Read the model definition and answer for the solid it produces. Units are mm, in the model's axes. A direction names the side the tool comes from. Give positions to 0.01 mm unless a question says otherwise; leave off trailing zeros. Return JSON: item names as keys, results as strings.
```python
from build123d import *
from OCP.BRepFilletAPI import BRepFilletAPI_MakeChamfer

# Parameters (mm, degrees)
BOSS_EXTRUDE1_DEPTH     = 27
SKETCH2_W               = 339
SKETCH2_H               = 271
CUT_EXTRUDE1_DEPTH      = 2.54
FILLET2_R               = 0.254
ESQUISSE1_W             = 314
ESQUISSE1_H             = 295.992698065
BOSS_EXTRU_1_DEPTH      = 25
CHANFREIN1_SIZE         = 25
CHANFREIN1_SIZE_2       = 35
ENL_V_MAT_EXTRU_1_DEPTH = 25
ESQUISSE3_R             = 2.5
ENL_V_MAT_EXTRU_2_DEPTH = 15


with BuildPart() as part:
    # Sketch1 → Boss-Extrude1 (new body)
    with BuildSketch(Plane.XY):
        with BuildLine():
            Line((9.729828387, -0.262968335), (184.729828387, -4.992698065))
            ThreePointArc((184.729828387, -4.992698065), (185, -4.996348366), (185.270171613, -4.992698065))
            Line((185.270171613, -4.992698065), (360.270171613, -0.262968335))
            ThreePointArc((360.270171613, -0.262968335), (367.165951302, 2.758487678), (370, 9.733381364))
            Line((370, 9.733381364), (370, 340))
            Line((370, 340), (0, 340))
            Line((0, 340), (0, 9.733381364))
            ThreePointArc((0, 9.733381364), (2.834048698, 2.758487678), (9.729828387, -0.262968335))
        make_face()
    extrude(amount=BOSS_EXTRUDE1_DEPTH)

    # Sketch2 → Cut-Extrude1 (cut)
    with BuildSketch(Plane.XY.offset(27)):
        with Locations((185, 184.5)):
            Rectangle(SKETCH2_W, SKETCH2_H)
    extrude(amount=-CUT_EXTRUDE1_DEPTH, mode=Mode.SUBTRACT)

    # Fillet2
    fillet2_edges = [part.edges().sort_by_distance(p)[0] for p in [
        (354.5, 184.5, 24.46),
        (15.5, 184.5, 27),
        (185, 49, 27),
        (185, 320, 27),
    ]]
    fillet(fillet2_edges, radius=FILLET2_R)

    # Esquisse1 → Boss.-Extru.1 (add)
    with BuildSketch(Plane(origin=(0, 0, 0), x_dir=(-1, 0, 0), z_dir=(0, 0, -1))):
        with Locations((-185, 155.003650967)):
            Rectangle(ESQUISSE1_W, ESQUISSE1_H)
    extrude(amount=BOSS_EXTRU_1_DEPTH)

    # Chanfrein1
    chanfrein1_edges_1 = [part.edges().sort_by_distance(p)[0] for p in [
        (28, 155.003650968, -25),
    ]]
    chanfrein1_side_1 = [part.faces().sort_by_distance(p)[0] for p in [
        (28, 155.003650968, -24.5),
    ]]
    chanfrein1_edges_2 = [part.edges().sort_by_distance(p)[0] for p in [
        (185, 303, -25),
    ]]
    chanfrein1_side_2 = [part.faces().sort_by_distance(p)[0] for p in [
        (185, 303, -24.5),
    ]]
    chanfrein1_edges_3 = [part.edges().sort_by_distance(p)[0] for p in [
        (342, 155.003650968, -25),
    ]]
    chanfrein1_side_3 = [part.faces().sort_by_distance(p)[0] for p in [
        (342, 155.003650968, -24.5),
    ]]
    chanfrein1 = BRepFilletAPI_MakeChamfer(part.part.solid().wrapped)
    for e in chanfrein1_edges_1:
        chanfrein1.Add(CHANFREIN1_SIZE - 0.0001, CHANFREIN1_SIZE_2 - 0.0001, e.wrapped, chanfrein1_side_1[0].wrapped)
    for e in chanfrein1_edges_2:
        chanfrein1.Add(CHANFREIN1_SIZE - 0.0001, CHANFREIN1_SIZE_2 - 0.0001, e.wrapped, chanfrein1_side_2[0].wrapped)
    for e in chanfrein1_edges_3:
        chanfrein1.Add(CHANFREIN1_SIZE - 0.0001, CHANFREIN1_SIZE_2 - 0.0001, e.wrapped, chanfrein1_side_3[0].wrapped)
    add(Compound.cast(chanfrein1.Shape()), mode=Mode.REPLACE)  # a hair under: the kernel refuses the full size

    # Esquisse2 → Enlèv. mat.-Extru.1 (cut)
    with BuildSketch(Plane(origin=(0, 0, -25), x_dir=(-1, 0, 0), z_dir=(0, 0, -1))):
        Polygon((-273.063305356, 7.007301935), (-89.826670404, 7.007301935), (-89.826670404, 60.007301935), (-66.826670404, 60.007301935), (-66.826670404, 108.007301935), (-296.063305356, 108.007301935), (-296.063305356, 60.007301935), (-273.063305356, 60.007301935), align=None)
    extrude(amount=-ENL_V_MAT_EXTRU_1_DEPTH, mode=Mode.SUBTRACT)

    # Esquisse3 → Enlèv. mat.-Extru.2 (cut)
    with BuildSketch(Plane(origin=(0, 0, -25), x_dir=(-1, 0, 0), z_dir=(0, 0, -1))):
        with Locations((-188, 255.8)):
            Circle(ESQUISSE3_R)
        with Locations((-238, 193)):
            Circle(ESQUISSE3_R)
        with Locations((-132, 193)):
            Circle(ESQUISSE3_R)
    extrude(amount=-ENL_V_MAT_EXTRU_2_DEPTH, mode=Mode.SUBTRACT)


solid = part.part
```
Q1. Consider L1, parallel to X at y = 193, z = -19.25; L2, parallel to X at y = 193, z = -19; L3, parallel to Y at x = 282, z = -19. Determine where each line is inside the solid, lowest interval first.
Values:
{"L1": "x = 54.95 to 129.5, 134.5 to 235.5, 240.5 to 315.05", "L2": "x = 54.6 to 129.5, 134.5 to 235.5, 240.5 to 315.4", "L3": "y = 7.01 to 60.01, 108.01 to 276.4"}
Q2. Determine the mould class of faces 5 (the flat face through (296.063, 84, -13)), 6 (the flat face through (300, 7.007, -12)), 7 (the flat face through (273.063, 34, -13)), 8 (the flat face through (183, 186, 24.46)) for opening direction Y: released by +Y, released by -Y, zero draft, split by the parting line, or undercut.
Values:
{"face 5": "undercut", "face 6": "released by -Y", "face 7": "zero draft", "face 8": "undercut"}
Q3. Given pin 1 (3 mm diameter, centred on x = 253, z = -18, fed in from +Y); pin 2 (3 mm diameter, centred on x = 187.5, z = -13, fed in from +Y); pin 3 (5 mm diameter, centred on x = 164.5, y = 305.5, fed in from +Z), each flat-ended and moving along its own axis, determine where each tip first touches the part or whether it passes through.
Values:
{"pin 1": "stops at y = 279.9", "pin 2": "stops at y = 286.9", "pin 3": "stops at z = 24.46"}
Q4. For faces 1 (the flat face through (66.827, 84, -13)), 2 (the flat face through (187.198, 285.255, -12.675)), 3 (the flat face through (89.827, 33, -13)), 4 (the flat face through (66, 7.007, -10)), determine the directions among +Z, -Z, +X, -X, +Y, -Y from which every point of the face is accessible in a straight line to the end or side of a thin tool.
Values:
{"face 1": "-Z", "face 2": "-Z, +X, -X, +Y", "face 3": "-Z, -Y", "face 4": "-Z, +X, -X, -Y"}
